Geometry check sheet. Reference: drawing and pictorial views, mm from the part's lowest x, y, z. A direction names the side the tool comes from. Give positions to 0.01 mm unless a question says otherwise; leave off trailing zeros. Loops run counter-clockwise (first coordinate to the right, second up) from the corner with the lowest first, then second, coordinate; pieces in that order, holes last. Notation, with made-up numbers: (60.25, -6.5) -> (81.25, -6.5) arc R31 ccw to (81.25, 20.5) -> close; hole circle Ø4 at (0, 54). An arc over 180 degrees is marked (long way). Write item = value, one per line. Start each with the question number.
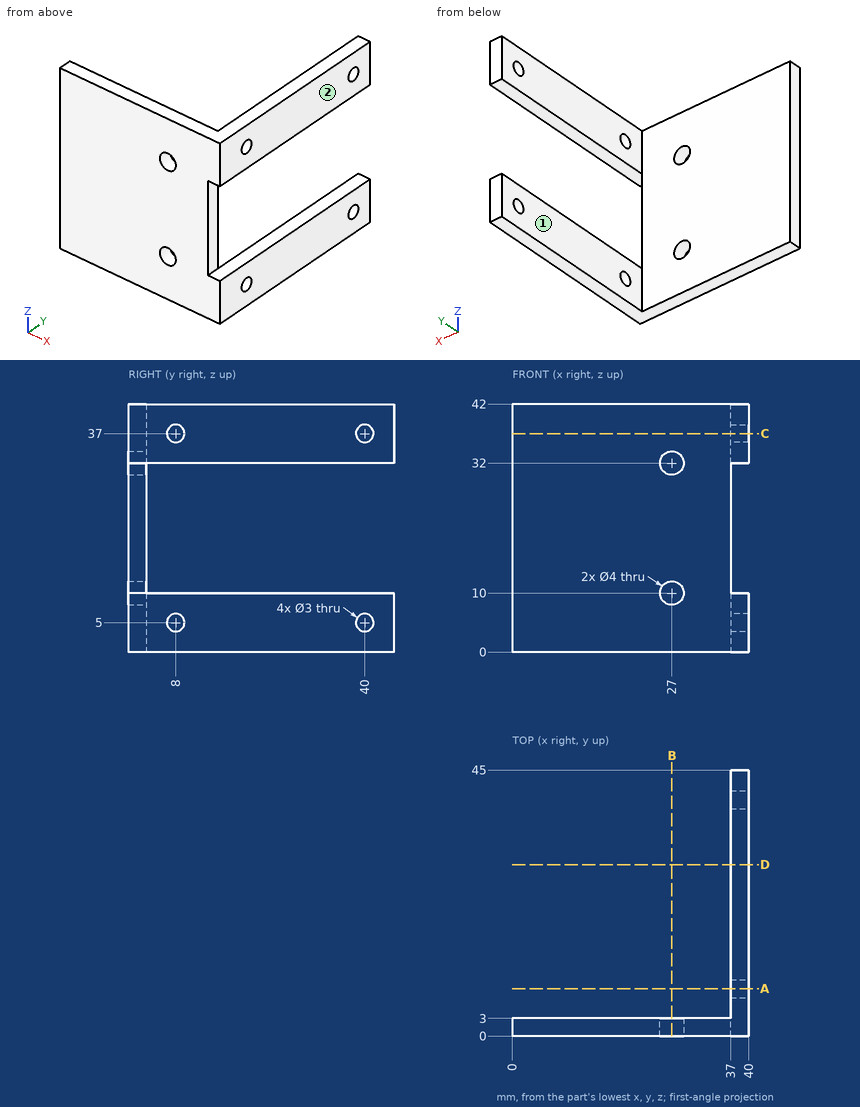
1) Section check A-A (y = 8). Enter the section's corners in (x, z), plus the area to 3 significant figures.
2) Section check D-D (y = 29). Enter the section's corners in (x, z).
3) Section check C-C (z = 37). Enter the section's corners in (x, y), plus the area to 3 significant figures.
4) Section check B-B (x = 27). Enter the section's corners in (y, z).
5) Depth check by flat-ended pin: pin 1 Ø8 at (y, z) = (23.5, 39.5) entering from -X; pin 2 Ø10 at (x, y) = (29.5, 12) entering from +Z; pin 3 Ø6 at (x, z) = (22, 5.5) entering from +Y; pin 4 Ø0.9 at (x, y) = (38.5, 14.5) entering from -Z. Enter the tip coordinate at first touch or a pass-through.
6) Tool access check on the marked faces 1 and 2. Record the directions out of +Z, -Z, +X, -X, +Y, -Y that give a thin tool (end or side, any length) a straight path to the whole face; none if there is none.
7) Thickness scan on line 1 (Y direction, x = 39.2, z = 5); line 2 (X direction, y = 19, z = 7); line 3 (Y direction, x = 20.5, z = 16). Record the ranges inside material, lowest first.
Check result:
q1.outline = (37, 0) -> (40, 0) -> (40, 3.5) -> (37, 3.5) -> close; (37, 6.5) -> (40, 6.5) -> (40, 10) -> (37, 10) -> close; (37, 32) -> (40, 32) -> (40, 35.5) -> (37, 35.5) -> close; (37, 38.5) -> (40, 38.5) -> (40, 42) -> (37, 42) -> close
q1.area = 42.0 mm2
q2.outline = (37, 0) -> (40, 0) -> (40, 10) -> (37, 10) -> close; (37, 32) -> (40, 32) -> (40, 42) -> (37, 42) -> close
q3.outline = (0, 0) -> (40, 0) -> (40, 6.5) -> (37, 6.5) -> (37, 3) -> (0, 3) -> close; (37, 9.5) -> (40, 9.5) -> (40, 38.5) -> (37, 38.5) -> close; (37, 41.5) -> (40, 41.5) -> (40, 45) -> (37, 45) -> close
q3.area = 228 mm2
q4.outline = (0, 0) -> (3, 0) -> (3, 8) -> (0, 8) -> close; (0, 12) -> (3, 12) -> (3, 30) -> (0, 30) -> close; (0, 34) -> (3, 34) -> (3, 42) -> (0, 42) -> close
q5.pin_1 = 37
q5.pin_2 = through
q5.pin_3 = 3
q5.pin_4 = 0
q6.face_1 = +Z, -Z, -X, +Y
q6.face_2 = +Z, -Z, +X, +Y, -Y
q7.line_1 = 0 to 6.5, 9.5 to 38.5, 41.5 to 45
q7.line_2 = 37 to 40
q7.line_3 = 0 to 3
